Read the model definition and answer for the solid it produces. Units are mm, in the model's axes. A direction names the side the tool comes from. Give positions to 0.01 mm unless a question says otherwise; leave off trailing zeros. Order: outer loops, then holes, each group sorted by start corner. A loop starts at its lowest first (then second) coordinate and runs counter-clockwise, first axis right, second up. Notation, with made-up numbers: (-5, 13) -> (24, 13) arc R34 ccw to (24, 44) -> close; hole circle Ø4 at (39, 65.25). An arc over 180 degrees is marked (long way). Answer as CSV lines item,"result". Start each with the question number.
1) Flat-ended cylindrical pins translate along their axes: pin 1 Ø1.5 at (x, z) = (11.5, 5) entering from -Y; pin 2 Ø0.7 at (x, y) = (3.5, 0) entering from -Z; pin 3 Ø0.9 at (x, z) = (-12.5, 5.5) entering from +Y. Find the tip coordinate at first contact, or state that the pin passes through.
2) Straight lines are drawn through the part: L1, parallel to Y at x = 4.25, z = 2; L2, parallel to X at y = 1, z = 9.25; L3, parallel to Y at x = -1.5, z = 3.5. For each, find the intervals that lie inside material, in ascending order. Write a range as from..to.
3) Find section C-C (z = 5.25). Determine the outline of the cut face in (x, y).
4) Find section A-A (z = 8). Determine the outline of the cut face in (x, y), and give its area (3 significant figures).
5) The mould has two halves that part along X. Classify faces 1 (the face through (7.25, 0, 5)), 2 (the face through (7.75, 0, 9)), 3 (the face through (-7.75, 0, 9)): +X half, -X half, draft (parallel to the pull), parting line (faces both ways), or undercut.
6) Find section D-D (x = 2). Determine the outline of the cut face in (y, z), and give its area (3 significant figures).
7) For faces 4 (the face through (-1, 4, 1)), 5 (the face through (-4, 0, 0.5)), 6 (the face through (-7.75, 0, 1)), 7 (the face through (6.76, 2.99, 9.22)), determine the directions among +Z, -Z, +X, -X, +Y, -Y from which every point of the face is accessible in a straight line to the end or side of a thin tool.
8) Find section B-B (y = 0). State how many separate pieces and enclosed holes the cut face has, and give its area (3 significant figures).
```python
from build123d import *

# Parameters (mm, degrees)
BOSS_EXTRUDE1_DEPTH = 11.5
SKETCH2_R           = 1.25
BOSS_EXTRUDE2_DEPTH = 4
BOSS_EXTRUDE3_DEPTH = 2
SKETCH4_R           = 1.139512492
SKETCH4_R_2         = 1.383403708
BOSS_EXTRUDE4_DEPTH = 9


with BuildPart() as part:
    # Sketch1 → Boss-Extrude1 (new body)
    with BuildSketch(Plane.XY):
        Polygon((5.75, -4), (7.75, -2), (7.75, 2), (5.75, 4), (-7.75, 4), (-7.75, -4), align=None)
        Polygon((-7.25, 3.5), (-7.25, -3.5), (5.542893219, -3.5), (7.25, -1.792893219), (7.25, 1.792893219), (5.542893219, 3.5), align=None, mode=Mode.SUBTRACT)
    extrude(amount=BOSS_EXTRUDE1_DEPTH)

    # Sketch2 → Boss-Extrude2 (add)
    with BuildSketch(Plane(origin=(0, 0, 3), x_dir=(-1, 0, 0), z_dir=(0, 0, -1))):
        Polygon((-13.5, 0), (-13.5, 4), (-10.5, 4), (-8.5, 6), (8.5, 6), (10.5, 4), (13.5, 4), (13.5, 0), (13.5, -4), (10.5, -4), (8.5, -6), (-8.5, -6), (-10.5, -4), (-13.5, -4), align=None)
        with Locations((-10.5, 0)):
            Circle(SKETCH2_R, mode=Mode.SUBTRACT)
        with Locations((10.5, 0)):
            Circle(SKETCH2_R, mode=Mode.SUBTRACT)
        Polygon((-5.75, -4), (7.75, -4), (7.75, 4), (-5.75, 4), (-7.75, 2), (-7.75, -2), align=None, mode=Mode.SUBTRACT)
    extrude(amount=-BOSS_EXTRUDE2_DEPTH)

    # Sketch3 → Boss-Extrude3 (add)
    with BuildSketch(Plane.XY.offset(11.5)):
        Polygon((-7.25, 3.5), (-7.25, -3.5), (5.542893219, -3.5), (7.25, -1.792893219), (7.25, 1.792893219), (5.542893219, 3.5), align=None)
    extrude(amount=-BOSS_EXTRUDE3_DEPTH)

    # Sketch4 → Boss-Extrude4 (add)
    with BuildSketch(Plane(origin=(0, 0, 9.5), x_dir=(-1, 0, 0), z_dir=(0, 0, -1))):
        with Locations(Location((-4.01250784, 0, 0), (0, 0, 180))):
            Circle(SKETCH4_R)
        with Locations(Location((3.818130298, 0, 0), (0, 0, 180))):
            Circle(SKETCH4_R_2)
    extrude(amount=BOSS_EXTRUDE4_DEPTH)


solid = part.part
```
Findings below:
1,pin 1,"y = -4"
1,pin 2,"z = 0.5"
1,pin 3,"y = 4"
2,L1,"-4..-3.5, -1.11..1.11, 3.5..4"
2,L2,"-7.75..-7.25, -4.77..-2.86, 3.47..4.56, 7.25..7.75"
2,L3,"-6..-3.5, 3.5..6"
3,outline,"(-13.5, -4) -> (-10.5, -4) -> (-8.5, -6) -> (8.5, -6) -> (10.5, -4) -> (13.5, -4) -> (13.5, 4) -> (10.5, 4) -> (8.5, 6) -> (-8.5, 6) -> (-10.5, 4) -> (-13.5, 4) -> close; circle Ø2.77 at (-3.82, 0); circle Ø2.28 at (4.01, 0); hole circle Ø2.5 at (-10.5, 0); hole (-7.25, -3.5) -> (5.54, -3.5) -> (7.25, -1.79) -> (7.25, 1.79) -> (5.54, 3.5) -> (-7.25, 3.5) -> close; hole circle Ø2.5 at (10.5, 0)"
4,outline,"(-7.75, -4) -> (5.75, -4) -> (7.75, -2) -> (7.75, 2) -> (5.75, 4) -> (-7.75, 4) -> close; circle Ø2.77 at (-3.82, 0); circle Ø2.28 at (4.01, 0); hole (-7.25, -3.5) -> (5.54, -3.5) -> (7.25, -1.79) -> (7.25, 1.79) -> (5.54, 3.5) -> (-7.25, 3.5) -> close"
4,area,"31.5 mm²"
5,face 1,"undercut"
5,face 2,"+X half"
5,face 3,"-X half"
6,outline,"(-6, 3) -> (-4, 3) -> (-4, 0) -> (-3.5, 0) -> (-3.5, 9.5) -> (3.5, 9.5) -> (3.5, 0) -> (4, 0) -> (4, 3) -> (6, 3) -> (6, 7) -> (4, 7) -> (4, 11.5) -> (-4, 11.5) -> (-4, 7) -> (-6, 7) -> close"
6,area,"41.5 mm²"
7,face 4,"-Z, +X, -X, +Y"
7,face 5,"-Z"
7,face 6,"-Z, -X, +Y, -Y"
7,face 7,"+Z, +X, +Y"
8,separate pieces,"3"
8,enclosed holes,"0"
8,area,"112 mm²"
